Here's how the part is built. I have some questions about the finished solid (model axes, mm). A direction names the side the tool comes from. Coordinates: 2 decimals unless noted, no trailing zeros. Write each loop counter-clockwise with the first axis right and the second up, starting at its lowest first coordinate (ties: lowest second). Pieces come first, ordered by that corner, then holes.
Item 1: I want a section at B-B (x = -24). Please give me the cut outline in (y, z).
Item 2: I want a section at D-D (y = 5.75). Please give me the cut outline in (x, z).
Item 3: If we mould it in two halves opening along Y, with no side actions, what happens to faces 1 (the face through (-4, 18.99, 27.04)), 2 (the face through (-25.22, 14.06, 5.61)), 3 (the face through (-25.09, 1.54, 13.42)), 4 (the face through (-27.64, 0.86, 23.1))? For each: pulls with the +Y half, pulls with the -Y half, needs draft (parallel to the pull), parting line crosses it, or undercut.
Item 4: For faces 5 (the face through (-28, 7, 24)), 6 (the face through (-34, 22, 13)), 7 (the face through (-26.36, 19.15, 20.99)), which set-ups out of +Z, -Z, +X, -X, +Y, -Y let a thin tool reach every point of the face, with its end or its side?
Item 5: I want a section at A-A (y = 11). Please give me the cut outline in (x, z).
Item 6: I want a section at C-C (y = 1.75). Please give me the cut outline in (x, z).
Item 7: Please list where these lines run through material, in increasing order: line 1 (Y direction, x = -21.5, z = 13); line 2 (Z direction, x = -6.5, y = 14.5); line 3 (Z direction, x = -7.5, y = 15.75).
Item 8: I'm going to push flat-ended pins straight in: P1, Ø4, axis at x = -20, z = 7, coming from the +Y side; P2, Ø9.5, axis at y = 11, z = 13, coming from the -X side; P3, Ø2.5, axis at x = -32, y = 5.5, coming from the +Z side. Where does each tip first touch, or does it pass through?
from build123d import *

# Parameters (mm, degrees)
BOSS_EXTRUDE3_DEPTH = 22
CUT_EXTRUDE4_DEPTH  = 59.108375
CUT_EXTRUDE5_REACH  = 125.396
SKETCH5_R           = 8
CUT_EXTRUDE6_REACH  = 125.396
SKETCH7_R           = 8
FILLET1_R           = 10
CUT_EXTRUDE9_DEPTH  = 28.41
CUT_EXTRUDE10_DEPTH = 33.85
BOSS_EXTRUDE4_REACH = 60.461
BOSS_EXTRUDE5_REACH = 60.461
BOSS_EXTRUDE6_REACH = 60.461
BOSS_EXTRUDE7_REACH = 60.461
CUT_EXTRUDE11_DEPTH = 40
FILLET2_R           = 3


with BuildPart() as part:
    # Sketch1 → Boss-Extrude3 (new body)
    with BuildSketch(Plane(origin=(0, 0, 0), x_dir=(1, 0, 0), z_dir=(0, 1, 0))):
        Polygon((36.111730264, -52.557630883), (46.787036785, -33.321263484), (-9.652310469, -2), (-68.760685704, -2), (-68.760685704, -24), (-15.347689531, -24), align=None)
    extrude(amount=BOSS_EXTRUDE3_DEPTH)

    # Sketch4 → Cut-Extrude4 (cut)
    with BuildSketch(Plane.ZY.offset(68.760685704)):
        with BuildLine():
            ThreePointArc((21, 11), (13, 19), (5, 11))
            Line((5, 11), (21, 11))
        make_face()
        with BuildLine():
            Line((21, 11), (5, 11))
            ThreePointArc((5, 11), (13, 3), (21, 11))
        make_face()
    extrude(amount=-CUT_EXTRUDE4_DEPTH, mode=Mode.SUBTRACT)

    # Cut-Extrude5: up to this plane
    cut_extrude5_end = Plane(origin=(-9.652310469, 0, 0), z_dir=(-1, 0, 0))
    # Sketch5 → Cut-Extrude5 (cut, up to the surface)
    with BuildSketch(Plane(origin=(49.908331158, 0, 27.696847436), x_dir=(0.4852412054872001, 0, -0.87438033629384), z_dir=(0.87438033629384, 0, 0.4852412054872001)), mode=Mode.PRIVATE) as cut_extrude5_sk1:
        with Locations((-17.43245944, 11)):
            Circle(SKETCH5_R)
    cut_extrude5_tool1 = split(extrude(cut_extrude5_sk1.sketch, amount=-CUT_EXTRUDE5_REACH, mode=Mode.PRIVATE), bisect_by=cut_extrude5_end, keep=Keep.BOTH, mode=Mode.PRIVATE)
    add(cut_extrude5_tool1.solids().sort_by_distance((41.449384, 11, 42.939447))[0], mode=Mode.SUBTRACT)

    # Sketch7 → Cut-Extrude6 (cut, up to next)
    with BuildSketch(Plane(origin=(49.908331158, 0, 27.696847436), x_dir=(0.4852412054872001, 0, -0.87438033629384), z_dir=(0.87438033629384, 0, 0.4852412054872001)), mode=Mode.PRIVATE) as cut_extrude6_sk1:
        with Locations((-17.43245944, 11)):
            Circle(SKETCH7_R)
    cut_extrude6_tool1 = extrude(cut_extrude6_sk1.sketch, amount=-CUT_EXTRUDE6_REACH, mode=Mode.PRIVATE) & part.part
    add(cut_extrude6_tool1.solids().sort_by_distance((41.449384, 11, 42.939447))[0], mode=Mode.SUBTRACT)

    # Fillet1
    fillet1_edges = [part.edges().sort_by_distance(p)[0] for p in [
        (18.567363158, 0, 17.660631742),
        (10.382020367, 0, 38.278815441),
        (18.567363158, 22, 17.660631742),
        (-39.206498086, 22, 2),
        (-42.054187617, 22, 24),
        (10.382020367, 22, 38.278815441),
        (-42.054187617, 0, 24),
        (-39.206498086, 0, 2),
    ]]
    fillet(fillet1_edges, radius=FILLET1_R)

    # Sketch9 → Cut-Extrude9 (cut)
    with BuildSketch(Plane.ZY.offset(68.760685704)):
        with BuildLine():
            Line((2, 12), (2, 10))
            ThreePointArc((2, 10), (4.928932188, 2.928932188), (12, 0))
            Line((12, 0), (14, 0))
            ThreePointArc((14, 0), (21.071067812, 2.928932188), (24, 10))
            Line((24, 10), (24, 12))
            ThreePointArc((24, 12), (21.071067812, 19.071067812), (14, 22))
            Line((14, 22), (12, 22))
            ThreePointArc((12, 22), (4.928932188, 19.071067812), (2, 12))
        make_face()
    extrude(amount=-CUT_EXTRUDE9_DEPTH, mode=Mode.SUBTRACT)

    # Sketch10 → Cut-Extrude10 (cut)
    with BuildSketch(Plane(origin=(49.908331158, 0, 27.696847436), x_dir=(0.4852412054872001, 0, -0.87438033629384), z_dir=(0.87438033629384, 0, 0.4852412054872001))):
        with BuildLine():
            Line((-18.43245944, 0), (-16.43245944, 0))
            ThreePointArc((-16.43245944, 0), (-9.361391629, 2.928932188), (-6.43245944, 10))
            Line((-6.43245944, 10), (-6.43245944, 12))
            ThreePointArc((-6.43245944, 12), (-9.361391629, 19.071067812), (-16.43245944, 22))
            Line((-16.43245944, 22), (-18.43245944, 22))
            ThreePointArc((-18.43245944, 22), (-25.503527252, 19.071067812), (-28.43245944, 12))
            Line((-28.43245944, 12), (-28.43245944, 10))
            ThreePointArc((-28.43245944, 10), (-25.503527252, 2.928932188), (-18.43245944, 0))
        make_face()
    extrude(amount=-CUT_EXTRUDE10_DEPTH, mode=Mode.SUBTRACT)

    # Sketch11 → Boss-Extrude4 (add, up to next)
    with BuildSketch(Plane.XZ, mode=Mode.PRIVATE) as boss_extrude4_sk1:
        Polygon((-15.347689531, 24), (-40.350685704, 24), (-40.350685704, 14), (-12.758880866, 14), align=None)
    boss_extrude4_tool1 = extrude(boss_extrude4_sk1.sketch, amount=-BOSS_EXTRUDE4_REACH, mode=Mode.PRIVATE) - part.part
    add(boss_extrude4_tool1.solids().sort_by_distance((-27.191367, 0, 18.917964))[0])

    # Sketch12 → Boss-Extrude5 (add, up to next)
    with BuildSketch(Plane.XZ, mode=Mode.PRIVATE) as boss_extrude5_sk1:
        Polygon((6.513955881, 36.132216077), (-15.347689531, 24), (-12.758880866, 14), (11.366367936, 27.388412714), align=None)
    boss_extrude5_tool1 = extrude(boss_extrude5_sk1.sketch, amount=-BOSS_EXTRUDE5_REACH, mode=Mode.PRIVATE) - part.part
    add(boss_extrude5_tool1.solids().sort_by_distance((-2.526039, 0, 25.303272))[0])

    # Sketch13 → Boss-Extrude6 (add, up to next)
    with BuildSketch(Plane.XZ, mode=Mode.PRIVATE) as boss_extrude6_sk1:
        Polygon((-40.350685704, 12), (-12.241119134, 12), (-9.652310469, 2), (-40.350685704, 2), align=None)
    boss_extrude6_tool1 = extrude(boss_extrude6_sk1.sketch, amount=-BOSS_EXTRUDE6_REACH, mode=Mode.PRIVATE) - part.part
    add(boss_extrude6_tool1.solids().sort_by_distance((-25.639203, 0, 6.926631))[0])

    # Sketch14 → Boss-Extrude7 (add, up to next)
    with BuildSketch(Plane.XZ, mode=Mode.PRIVATE) as boss_extrude7_sk1:
        Polygon((-12.241119134, 12), (12.336850347, 25.639652042), (17.189262401, 16.895848679), (-9.652310469, 2), align=None)
    boss_extrude7_tool1 = extrude(boss_extrude7_sk1.sketch, amount=-BOSS_EXTRUDE7_REACH, mode=Mode.PRIVATE) - part.part
    add(boss_extrude7_tool1.solids().sort_by_distance((1.935469, 0, 14.065113))[0])

    # Sketch15 → Cut-Extrude11 (cut)
    with BuildSketch(Plane.XZ):
        with BuildLine():
            ThreePointArc((-27.825342852, 13), (-26.425342852, 11.6), (-25.025342852, 13))
            Line((-25.025342852, 13), (-27.825342852, 13))
        make_face()
        with BuildLine():
            Line((-27.825342852, 13), (-25.025342852, 13))
            ThreePointArc((-25.025342852, 13), (-26.425342852, 14.4), (-27.825342852, 13))
        make_face()
        with BuildLine():
            ThreePointArc((0.899937041, 20.436353877), (-1.003533117, 20.98114866), (-1.5483279, 19.077678501))
            Line((-1.5483279, 19.077678501), (0.899937041, 20.436353877))
        make_face()
        with BuildLine():
            Line((0.899937041, 20.436353877), (-1.5483279, 19.077678501))
            ThreePointArc((-1.5483279, 19.077678501), (0.026671027, 18.401696031), (1.075804571, 19.757016189))
            ThreePointArc((1.075804571, 19.757016189), (1.031124728, 20.107882646), (0.899937041, 20.436353877))
        make_face()
    extrude(amount=-CUT_EXTRUDE11_DEPTH, mode=Mode.SUBTRACT)

    # Fillet2
    fillet2_edges = [part.edges().sort_by_distance(p)[0] for p in [
        (-27.849187617, 0, 24),
        (-4.416866825, 0, 30.066108039),
        (-25.001498086, 0, 2),
        (3.768475966, 0, 9.447924339),
    ]]
    fillet(fillet2_edges, radius=FILLET2_R)


solid = part.part
Answer:
1. outline: (0, 5) arc R3 ccw to (3, 2) - (12, 2) arc R10 ccw to (22, 12) - (22, 14) arc R10 ccw to (12, 24) - (3, 24) arc R3 ccw to (0, 21) - close; hole circle Ø16 at (11, 13)
2. outline: (-40.35, 2) - (-9.65, 2) - (17.19, 16.9) - (14.78, 21.24) - (-9.65, 7.68) - (-9.65, 6.96) - (-40.35, 6.96) - close; (-40.35, 19.04) - (-14.06, 19.04) - (8.92, 31.79) - (6.51, 36.13) - (-15.35, 24) - (-40.35, 24) - close
3. face 1: pulls with the +Y half
3. face 2: undercut
3. face 3: needs draft
3. face 4: pulls with the -Y half
4. face 5: +Z, -X, +Y, -Y
4. face 6: +Z, -Z, +X, -X, +Y
4. face 7: +Z, -X, +Y
5. outline: (-40.35, 2) - (-9.65, 2) - (17.19, 16.9) - (15.73, 19.52) - (-9.65, 5.43) - (-9.65, 5) - (-40.35, 5) - close; (-40.35, 21) - (-14.57, 21) - (7.97, 33.51) - (6.51, 36.13) - (-15.35, 24) - (-40.35, 24) - close
6. outline: (-40.35, 2.27) - (-9.72, 2.27) - (17.06, 17.13) - (6.65, 35.89) - (-15.28, 23.73) - (-40.35, 23.73) - close; hole circle Ø2.8 at (-26.43, 13); hole circle Ø2.8 at (-0.32, 19.76)
7. line 1: y = 0 to 3, 19 to 22
7. line 2: z = 4.11 to 8.1, 24.56 to 28.55
7. line 3: z = 4.03 to 8.41, 23.14 to 27.52
8. P1: stops at y = 21.54
8. P2: stops at x = -4.57
8. P3: stops at z = 24
